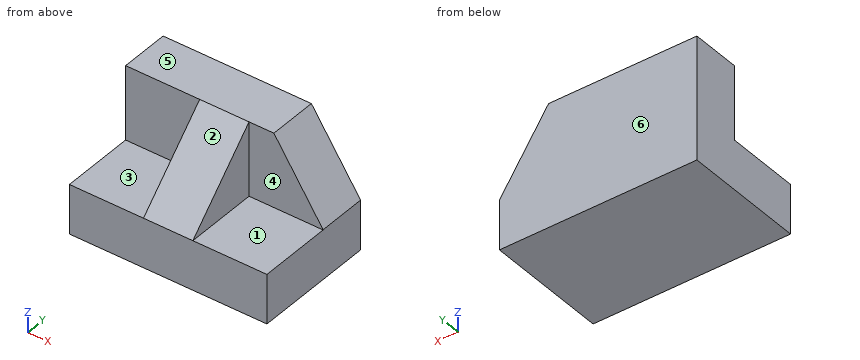
from build123d import *

# Parameters (mm, degrees)
F1_DEPTH = 50.8
F3_DEPTH = 31.75
F4_W     = 12.7
F4_H     = 19.05
F5_DEPTH = 31.75
F7_DEPTH = 25.4


with BuildPart() as f1:
    # F0 (on Right) → F1 (new body)
    with BuildSketch(Plane.YZ):
        Polygon((0, 12.7), (0, 0), (31.75, 0), (31.75, 31.75), (19.05, 31.75), (19.05, 12.7), align=None)
    extrude(amount=F1_DEPTH)

    # F2 (on Front) → F3 (cut)
    with BuildSketch(Plane.XZ):
        Polygon((50.8, 12.760184), (50.8, 31.810184), (38.1, 31.810184), align=None)
    extrude(amount=-F3_DEPTH, mode=Mode.SUBTRACT)

    # F4 (on Top) → F5 (join)
    with BuildSketch(Plane.XY):
        with Locations((25.4, 9.525)):
            Rectangle(F4_W, F4_H)
    extrude(amount=F5_DEPTH)

    # F6 (on face) → F7 (cut)
    with BuildSketch(Plane.YZ.offset(31.75)):
        Polygon((0, 12.7), (19.05, 31.75), (0, 31.75), align=None)
    extrude(amount=-F7_DEPTH, mode=Mode.SUBTRACT)


solid = f1.part
Work out the finished part from the listing and answer in its coordinate system (mm). Face numbers are marked on the shaded views. A direction names the side the tool comes from. Round coordinates to 2 decimals unless told otherwise and drop trailing zeros. Order: outer loops, then holes, each group sorted by start corner. A loop starts at its lowest first (then second) coordinate and runs counter-clockwise, first axis right, second up. Notation, with made-up numbers: M 56,1 L 110,1 A11 cw 110,15 Z; hole C 50.5,-12.5 d7. An arc over 180 degrees is marked long. Put each result on its own line as item: value. Start each with the question number.
Q1. Section B-B, the plane x = 24 is taken. Write down the section's boundary in (y, z).
Q2. Flat-ended cylindrical pins translate along their axes: pin 1 (15 mm diameter, centred on x = 9, y = 11, fed in from +Z); pin 2 (3 mm diameter, centred on y = 17, z = 26, fed in from -X); pin 3 (9.5 mm diameter, centred on x = 11.5, z = 17.5, fed in from -Y). Find the tip coordinate at first contact, or state that the pin passes through.
Q3. For a pull along Y with two mould halves and no side action, classify the marked faces 4, 5 and 6 as pulls with the +Y half, pulls with the -Y half, needs draft (parallel to the pull), parting line crosses it, or undercut.
Q4. Section C-C, the plane z = 13.5 is taken. Write down the section's boundary in (x, y), and give its area (3 significant figures).
Q5. Section A-A, the plane y = 13 is taken. Write down the section's boundary in (x, z).
Q6. A tool of negligible diameter and unlimited length cuts with its end or side. For the marked faces 1, 2 and 3, from which of +Z, -Z, +X, -X, +Y, -Y can it reach the whole face along a straight path? Write none if from no direction.
Q7. Section D-D, the plane y = 23 is taken. Write down the section's boundary in (x, z), and give its area (3 significant figures).
Q8. Straight lines are drawn through the part: L1, parallel to Z at x = 15, y = 5; L2, parallel to Y at x = 13, z = 13. For each, find the intervals that lie inside material, in ascending order. Write a range as [from, to].
Findings below:
1. outline: M 0,0 L 31.75,0 L 31.75,31.75 L 19.05,31.75 L 0,12.7 Z
2. pin 1: stops at z = 12.7
2. pin 2: stops at x = 19.05
2. pin 3: stops at y = 19.05
3. face 4: pulls with the -Y half
3. face 5: needs draft
3. face 6: pulls with the +Y half
4. outline: M 0,19.05 L 19.05,19.05 L 19.05,0.8 L 31.75,0.8 L 31.75,19.05 L 50.31,19.05 L 50.31,31.75 L 0,31.75 Z
4. area: 871 mm^2
5. outline: M 0,0 L 50.8,0 L 50.8,12.7 L 31.75,12.7 L 31.75,25.7 L 19.05,25.7 L 19.05,12.7 L 0,12.7 Z
6. face 1: +Z, +X, -Y
6. face 2: +Z, +X, -X, -Y
6. face 3: +Z, -X, -Y
7. outline: M 0,0 L 50.8,0 L 50.8,12.76 L 38.14,31.75 L 0,31.75 Z
7. area: 1,490 mm^2
8. L1: z = [0, 12.7]
8. L2: y = [19.05, 31.75]
